Geometry check sheet. Reference: drawing and pictorial views, mm from the part's lowest x, y, z. A direction names the side the tool comes from. Give positions to 0.01 mm unless a question says otherwise; leave off trailing zeros. Order: outer loops, then holes, each group sorted by start corner. A loop starts at its lowest first (then second) coordinate and runs counter-clockwise, first axis right, second up. Notation, with made-up numbers: M -13,49.5 L 29,49.5 A7 cw 29,56.5 Z; hole C 80,57 d1. An arc over 180 degrees is marked long. Answer as CSV lines item,"result".
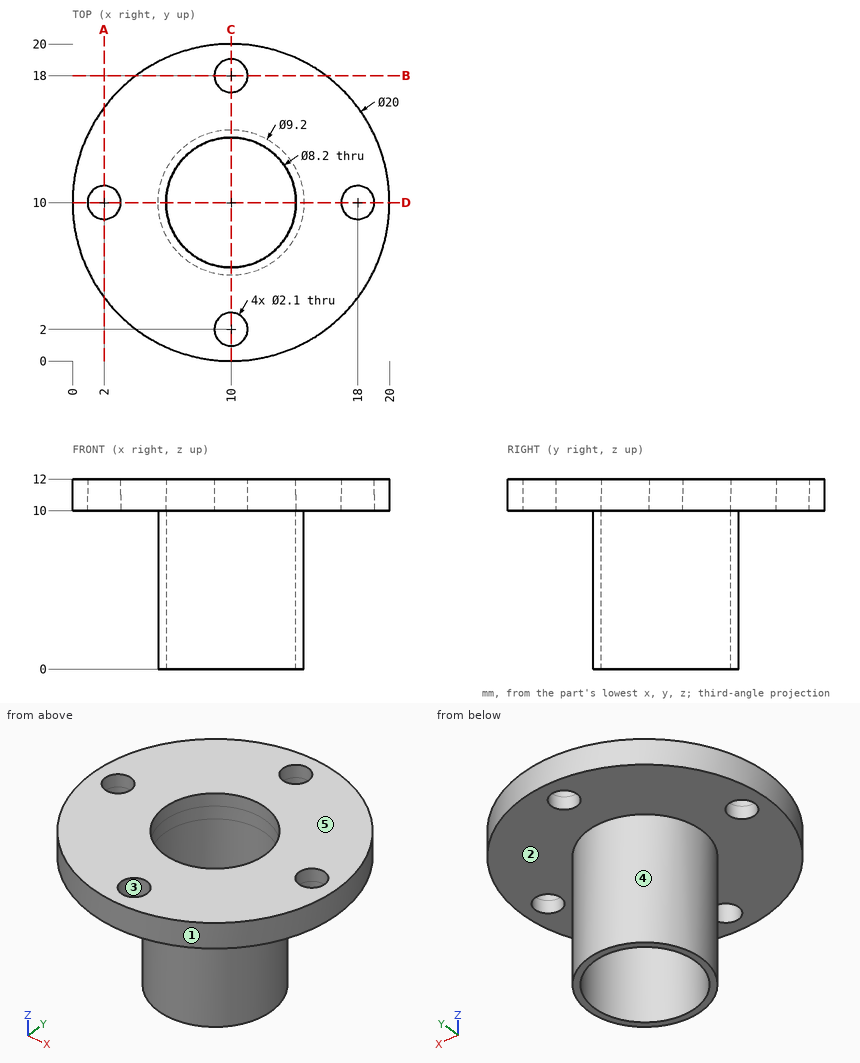
(1) Gauge pin test, flat ends, axial feed: P1, Ø3, axis at x = 6.5, y = 16.5, coming from the -Z side; P2, Ø5, axis at x = 12, z = 4, coming from the +Y side; P3, Ø4, axis at y = 13.5, z = 5, coming from the +X side. Record the tip position at first contact, or that the pin passes through.
The answers:
P1,"stops at z = 10"
P2,"stops at y = 14.6"
P3,"stops at x = 14.35"
(2) Draft check along X on the marked faces 3, 4 and 5. Enter one of: +X half, -X half, draft (parallel to the pull), parting line (faces both ways), or undercut.
The answers:
face 3,"undercut"
face 4,"parting line"
face 5,"draft"
(3) Section check A-A on x = 2. Enter the section's corners in (y, z).
The answers:
outline,"M 4,10 L 8.95,10 L 8.95,12 L 4,12 Z; M 11.05,10 L 16,10 L 16,12 L 11.05,12 Z"
(4) Tool access check on the marked faces 1 and 2. Record the directions out of +Z, -Z, +X, -X, +Y, -Y that give a thin tool (end or side, any length) a straight path to the whole face; none if there is none.
The answers:
face 1,"+Z, -Z"
face 2,"-Z"
(5) Material ranges on line 1 (Y direction, x = 10, z = 11.7); line 2 (Y direction, x = 18, z = 11.65); line 3 (Z direction, x = 11.25, y = 17), recorded low to high.
The answers:
line 1,"y = 0 to 0.95, 3.05 to 5.9, 14.1 to 16.95, 19.05 to 20"
line 2,"y = 4 to 8.95, 11.05 to 16"
line 3,"z = 10 to 12"
(6) Section check C-C on x = 10. Enter the section's corners in (y, z).
The answers:
outline,"M 0,10 L 0.95,10 L 0.95,12 L 0,12 Z; M 3.05,10 L 5.4,10 L 5.4,0 L 5.9,0 L 5.9,12 L 3.05,12 Z; M 14.1,0 L 14.6,0 L 14.6,10 L 16.95,10 L 16.95,12 L 14.1,12 Z; M 19.05,10 L 20,10 L 20,12 L 19.05,12 Z"
